from build123d import *

# Parameters (mm, degrees)
SKETCH_1_W          = 40
SKETCH_1_H          = 69.282032302
EXTRUDE_1_DEPTH     = 12
SKETCH_2_R          = 2.5
SKETCH_2_W          = 12
SKETCH_2_H          = 9.282032302
CUT_EXTRUDE_1_DEPTH = 12
SKETCH_3_R          = 2.5
CUT_EXTRUDE_2_DEPTH = 60
SKETCH_4_R          = 2.5
CUT_EXTRUDE_3_DEPTH = 12
SKETCH_5_R          = 4.5
CUT_EXTRUDE_4_DEPTH = 3
SKETCH_6_R          = 2.5
CUT_EXTRUDE_5_DEPTH = 10


with BuildPart() as part:
    # 草图1 → 凸台-拉伸1 (new body)
    with BuildSketch(Plane.XY):
        Rectangle(SKETCH_1_W, SKETCH_1_H)
    extrude(amount=EXTRUDE_1_DEPTH)

    # 草图2 → 切除-拉伸1 (cut)
    with BuildSketch(Plane.XY.offset(12)):
        with Locations((0, -30)):
            Circle(SKETCH_2_R)
        with Locations((0, 30)):
            Rectangle(SKETCH_2_W, SKETCH_2_H)
    extrude(amount=-CUT_EXTRUDE_1_DEPTH, mode=Mode.SUBTRACT)

    # 草图3 → 切除-拉伸2 (cut)
    with BuildSketch(Plane.ZY.offset(20)):
        with Locations((5, 30)):
            Circle(SKETCH_3_R)
    extrude(amount=-CUT_EXTRUDE_2_DEPTH, mode=Mode.SUBTRACT)

    # 草图4 → 切除-拉伸3 (cut)
    with BuildSketch(Plane(origin=(0, 0, 0), x_dir=(-1, 0, 0), z_dir=(0, 0, -1))):
        with Locations((-12, -9.641016151)):
            Circle(SKETCH_4_R)
        with Locations((-12, 5.358983849)):
            Circle(SKETCH_4_R)
        with Locations((-12, 20.358983849)):
            Circle(SKETCH_4_R)
        with Locations(Location((12, 20.358983849, 0), (0, 0, 180))):
            Circle(SKETCH_4_R)
        with Locations(Location((12, 5.358983849, 0), (0, 0, 180))):
            Circle(SKETCH_4_R)
        with Locations(Location((12, -9.641016151, 0), (0, 0, 180))):
            Circle(SKETCH_4_R)
    extrude(amount=-CUT_EXTRUDE_3_DEPTH, mode=Mode.SUBTRACT)

    # 草图5 → 切除-拉伸4 (cut)
    with BuildSketch(Plane(origin=(0, 0, 0), x_dir=(-1, 0, 0), z_dir=(0, 0, -1))):
        with Locations((-12, -9.641016151)):
            Circle(SKETCH_5_R)
        with Locations((-12, 5.358983849)):
            Circle(SKETCH_5_R)
        with Locations((-12, 20.358983849)):
            Circle(SKETCH_5_R)
        with Locations((12, -9.641016151)):
            Circle(SKETCH_5_R)
        with Locations((12, 5.358983849)):
            Circle(SKETCH_5_R)
        with Locations((12, 20.358983849)):
            Circle(SKETCH_5_R)
    extrude(amount=-CUT_EXTRUDE_4_DEPTH, mode=Mode.SUBTRACT)

    # 草图6 → 切除-拉伸5 (cut)
    with BuildSketch(Plane.XZ.offset(34.641016151)):
        with Locations(Location((-10, 6, 0), (0, 0, 270))):
            Circle(SKETCH_6_R)
        with Locations(Location((10, 6, 0), (0, 0, 270))):
            Circle(SKETCH_6_R)
    extrude(amount=-CUT_EXTRUDE_5_DEPTH, mode=Mode.SUBTRACT)


solid = part.part
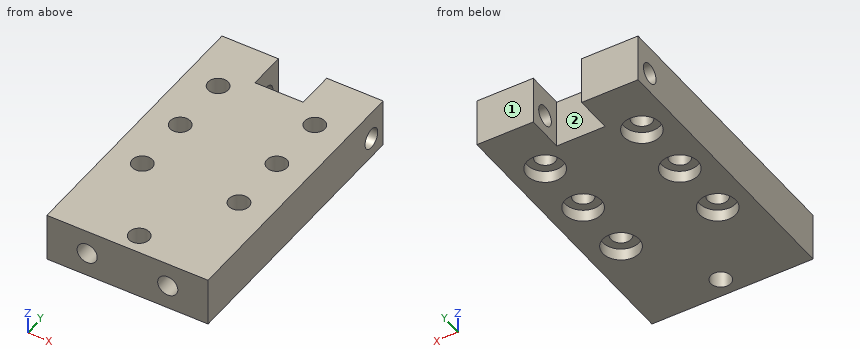
Work out the finished part from the listing and answer in its coordinate system (mm). Face numbers are marked on the shaded views. A direction names the side the tool comes from. Coordinates: 2 decimals unless noted, no trailing zeros. Write each loop counter-clockwise with the first axis right and the second up, starting at its lowest first coordinate (ties: lowest second). Pieces come first, ordered by that corner, then holes. Notation, with made-up numbers: M -12,-29.75 L 37,-29.75 A16 cw 37,-18.75 Z; hole C -16.5,-28.75 d2. An arc over 180 degrees is marked long. Use one line per item in the form item = value. Start each with the question number.
1. The part is cut by section B-B (x = 11). Give the number of separate pieces and of enclosed holes in the cut face, plus the area to 3 significant figures.
2. Straight lines are drawn through the part: probe 1 along X at (y, z) = (-27, 6.25); probe 2 along Y at (x, z) = (12.5, 10.25); probe 3 along X at (y, z) = (19.5, 8.75). For each, find the intervals that lie inside material, in ascending order. Write a range as from..to.
3. Each of these flat-tipped pins is pushed along its axis until it touches: P1, Ø4.5, axis at x = 12, y = -11, coming from the -Z side; P2, Ø1.5, axis at x = -9, z = 6, coming from the -Y side; P3, Ø4.5, axis at x = 12, y = -9.64, coming from the -Z side. Where does it stop, or does it pass through?
4. The part is cut by section A-A (y = -28.5). Give the vertices of the cut face in (x, z), plus the area to 3 significant figures.
5. A tool of negligible diameter and unlimited length cuts with its end or side. For the marked faces 1 and 2, from which of +Z, -Z, +X, -X, +Y, -Y can it reach the whole face along a straight path? Write none if from no direction.
6. The part is cut by section D-D (x = 0). Give the vertices of the cut face in (y, z), plus the area to 3 significant figures.
Evaluation:
q1.separate_pieces = 4
q1.enclosed_holes = 1
q1.area = 563 mm^2
q2.probe_1 = -20..-12.49, -7.51..7.51, 12.49..20
q2.probe_2 = -34.64..-12.09, -7.19..2.91, 7.81..17.91, 22.81..34.64
q2.probe_3 = -20..-14.35, -9.65..9.65, 14.35..20
q3.P1 = 3
q3.P2 = -24.64
q3.P3 = through
q4.outline = M -20,0 L -2,0 L -2,12 L -20,12 Z; M 2,0 L 20,0 L 20,12 L 2,12 Z; hole C -10,6 d5; hole C 10,6 d5
q4.area = 393 mm^2
q5.face_1 = +Z, -Z, +X, -X, +Y
q5.face_2 = +Z, -Z, +Y
q6.outline = M -34.64,0 L -32.5,0 L -32.5,12 L -34.64,12 Z; M -27.5,0 L 25.36,0 L 25.36,12 L -27.5,12 Z
q6.area = 660 mm^2
